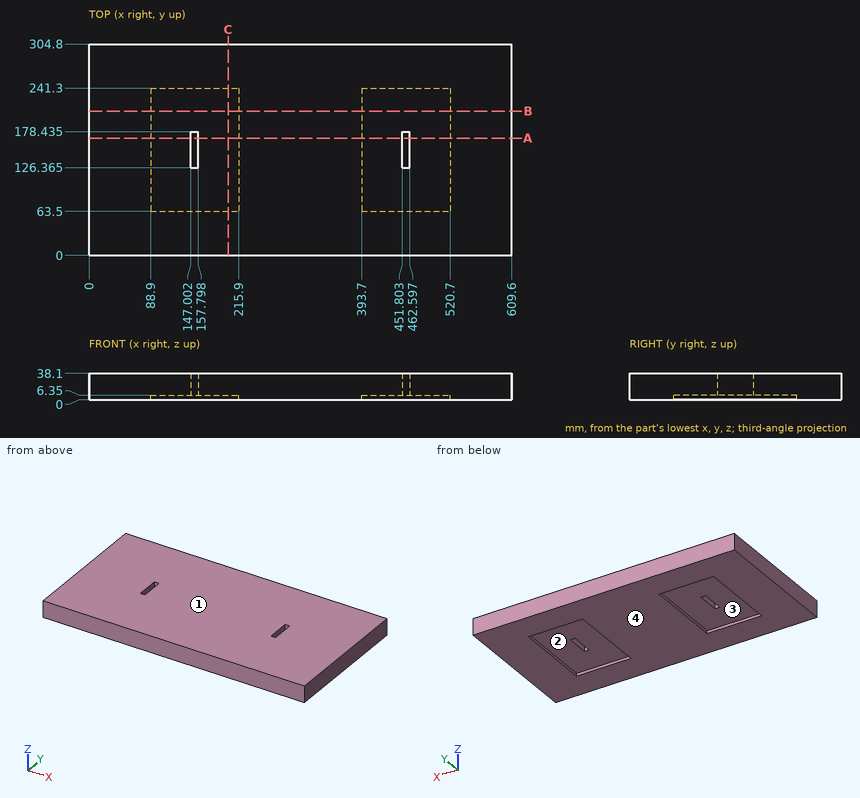
The figure shows three views and two pictorial views of one solid part (mm, origin at its lowest corner). Answer the questions. A direction names the side the tool comes from. Give positions to 0.01 mm unless a question says otherwise; leave off trailing zeros. Order: outer loops, then holes, each group sorted by start corner. A loop starts at its lowest first (then second) coordinate and runs counter-clockwise, first axis right, second up. Notation, with made-up numbers: (27.25, -27) -> (81.25, -27) arc R15 cw to (81.25, 0) -> close; hole circle Ø4 at (-29, 64). An arc over 180 degrees is marked (long way). Answer as a JSON object with one key per item and string values. Group by question number.
Item 1: The part is cut by section A-A on y = 169. Write down the section's boundary in (x, z), and give its area (3 significant figures).
Item 2: Consider L1, parallel to X at y = 131, z = 10; L2, parallel to Y at x = 486.5, z = 5; L3, parallel to Z at x = 435, y = 81.5. Determine where each line is inside the solid, lowest interval first. Write a range as from..to.
Item 3: A flat-ended cylindrical pin translates along its axis: pin 1 (4 mm diameter, centred on x = 123.5, y = 149, fed in from -Z). Find the tip coordinate at first contact, or state that the pin passes through.
Item 4: The part is cut by section C-C on x = 200.5. Write down the section's boundary in (y, z).
Item 5: The part is cut by section B-B on y = 208. Write down the section's boundary in (x, z), and give its area (3 significant figures).
Item 6: Determine the mould class of the marked faces 3 and 4 for opening direction Y: pulls with the +Y half, pulls with the -Y half, needs draft (parallel to the pull), parting line crosses it, or undercut.
Item 7: A tool of negligible diameter and unlimited length cuts with its end or side. For the marked faces 1 and 2, from which of +Z, -Z, +X, -X, +Y, -Y can it reach the whole face along a straight path? Write none if from no direction.
Result set:
{
 "1": {"outline": "(0, 0) -> (88.9, 0) -> (88.9, 6.35) -> (147, 6.35) -> (147, 38.1) -> (0, 38.1) -> close; (157.8, 6.35) -> (215.9, 6.35) -> (215.9, 0) -> (393.7, 0) -> (393.7, 6.35) -> (451.8, 6.35) -> (451.8, 38.1) -> (157.8, 38.1) -> close; (462.6, 6.35) -> (520.7, 6.35) -> (520.7, 0) -> (609.6, 0) -> (609.6, 38.1) -> (462.6, 38.1) -> close", "area": "20,900 mm²"},
 "2": {"L1": "0..147, 157.8..451.8, 462.6..609.6", "L2": "0..63.5, 241.3..304.8", "L3": "6.35..38.1"},
 "3": {"pin 1": "z = 6.35"},
 "4": {"outline": "(0, 0) -> (63.5, 0) -> (63.5, 6.35) -> (241.3, 6.35) -> (241.3, 0) -> (304.8, 0) -> (304.8, 38.1) -> (0, 38.1) -> close"},
 "5": {"outline": "(0, 0) -> (88.9, 0) -> (88.9, 6.35) -> (215.9, 6.35) -> (215.9, 0) -> (393.7, 0) -> (393.7, 6.35) -> (520.7, 6.35) -> (520.7, 0) -> (609.6, 0) -> (609.6, 38.1) -> (0, 38.1) -> close", "area": "21,600 mm²"},
 "6": {"face 3": "undercut", "face 4": "needs draft"},
 "7": {"face 1": "+Z, +X, -X, +Y, -Y", "face 2": "-Z"}
}
